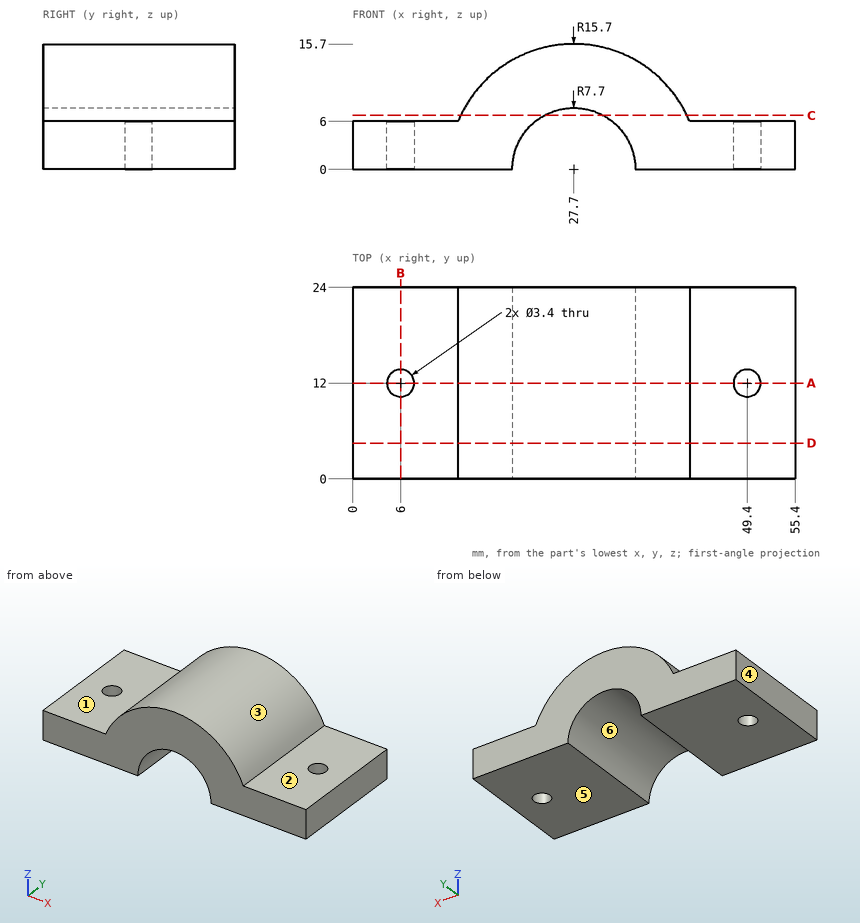
Source: three-view drawing plus pictorial views. Frame: mm from the lowest corner of the part. A direction names the side the tool comes from. Round coordinates to 2 decimals unless told otherwise and drop trailing zeros. Loops run counter-clockwise (first coordinate to the right, second up) from the corner with the lowest first, then second, coordinate; pieces in that order, holes last.
Q1. Section B-B, the plane x = 6. Return loops of the section in (y, z), plus the area to 3 significant figures.
Q2. Section A-A, the plane y = 12. Return loops of the section in (x, z), plus the area to 3 significant figures.
Q3. First-contact query: P1, Ø10.5, axis at x = 48.5, y = 9, coming from the +Z side; P2, Ø8, axis at y = 18.5, z = 12, coming from the -X side; P3, Ø1, axis at x = 40, y = 13.5, coming from the +Z side. Flat tips, straight axial feed; report the tip coordinate or a pass-through.
Q4. Mould query, pull axis X, two halves, no side actions, for the marked faces 4, 5 and 6. Classes: pulls with the +X half, pulls with the -X half, needs draft (parallel to the pull), parting line crosses it, or undercut.
Q5. Section D-D, the plane y = 4.5. Return loops of the section in (x, z).
Q6. Section C-C, the plane z = 6.75. Return loops of the section in (x, y), plus the area to 3 significant figures.
Q7. Ray query, line 1 (Y direction, x = 49.4, z = 1.25); line 2 (X direction, y = 13, z = 4); line 3 (X direction, y = 22, z = 1). Return the intervals inside material, ascending.
Q8. Access query for the marked faces 1, 2 and 3. Directions: +Z, -Z, +X, -X, +Y, -Y. A direction counts if a zero-diameter tool reaches every point of the face in a straight line with its end or side. Return the directions, or none.
Solutions:
1. outline: (0, 0) - (10.3, 0) - (10.3, 6) - (0, 6) - close; (13.7, 0) - (24, 0) - (24, 6) - (13.7, 6) - close
1. area: 124 mm2
2. outline: (0, 0) - (4.3, 0) - (4.3, 6) - (0, 6) - close; (7.7, 0) - (20, 0) arc R7.7 cw to (35.4, 0) - (47.7, 0) - (47.7, 6) - (42.21, 6) arc R15.7 ccw to (13.19, 6) - (7.7, 6) - close; (51.1, 0) - (55.4, 0) - (55.4, 6) - (51.1, 6) - close
2. area: 402 mm2
3. P1: stops at z = 6
3. P2: stops at x = 14.19
3. P3: stops at z = 10.36
4. face 4: pulls with the -X half
4. face 5: needs draft
4. face 6: undercut
5. outline: (0, 0) - (20, 0) arc R7.7 cw to (35.4, 0) - (55.4, 0) - (55.4, 6) - (42.21, 6) arc R15.7 ccw to (13.19, 6) - (0, 6) - close
6. outline: (13.53, 0) - (23.99, 0) - (23.99, 24) - (13.53, 24) - close; (31.41, 0) - (41.87, 0) - (41.87, 24) - (31.41, 24) - close
6. area: 503 mm2
7. line 1: y = 0 to 10.3, 13.7 to 24
7. line 2: x = 0 to 4.63, 7.37 to 21.12, 34.28 to 48.03, 50.77 to 55.4
7. line 3: x = 0 to 20.07, 35.33 to 55.4
8. face 1: +Z, -X, +Y, -Y
8. face 2: +Z, +X, +Y, -Y
8. face 3: +Z, +Y, -Y
